Design review of the part built by this model. Coordinates are the model's own, in mm. Face numbers are marked on the shaded views. A direction names the side the tool comes from. Coordinates: 2 decimals unless noted, no trailing zeros. Loops run counter-clockwise (first coordinate to the right, second up) from the corner with the lowest first, then second, coordinate; pieces in that order, holes last. Notation, with made-up numbers: (-39, -14) -> (-15, -14) arc R5 ccw to (-15, -8) -> close; hole circle Ø1 at (34, 28.25). An arc over 180 degrees is marked (long way). Use CSV: the item, a comma, the result in double quotes.
```python
from build123d import *

# Parameters (mm, degrees)
ESQUISSE1_R                  = 4.25
ESQUISSE1_R_2                = 1.7
BOSS_EXTRU_1_DEPTH           = 5
ESQUISSE2_R                  = 3
ENL_V_MAT_EXTRU_1_DEPTH      = 3
BOSS_EXTRU_2_DEPTH           = 3
R_P_TITION_CIRCULAIRE1_DEPTH = 4
ESQUISSE4_R                  = 1
BOSS_EXTRU_3_DEPTH           = 2
R_P_TITION_CIRCULAIRE2_COUNT = 6
ENL_V_START                  = -1
ESQUISSE5_R                  = 3
ENL_V_MAT_EXTRU_2_DEPTH      = 1
CONG_1_R                     = 0.2
ESQUISSE6_R                  = 4.5
ESQUISSE6_R_2                = 3.5
ENL_V_MAT_EXTRU_3_DEPTH      = 1
CONG_2_R                     = 0.25
SCALE1_SCALE                 = 1.05


with BuildPart() as part:
    # Esquisse1 → Boss.-Extru.1 (new body)
    with BuildSketch(Plane.XY):
        Circle(ESQUISSE1_R)
        Circle(ESQUISSE1_R_2, mode=Mode.SUBTRACT)
    extrude(amount=BOSS_EXTRU_1_DEPTH)

    # Esquisse2 → Enlèv. mat.-Extru.1 (cut)
    with BuildSketch(Plane(origin=(0, 0, 0), x_dir=(-1, 0, 0), z_dir=(0, 0, -1))):
        Circle(ESQUISSE2_R)
    extrude(amount=-ENL_V_MAT_EXTRU_1_DEPTH, mode=Mode.SUBTRACT)

    # Esquisse3 → Boss.-Extru.2 (add)
    with BuildSketch(Plane(origin=(0, 0, 0), x_dir=(-1, 0, 0), z_dir=(0, 0, -1))):
        Polygon((-0.3, 3), (0, 2.6), (0.3, 3), align=None)
    extrude(amount=-BOSS_EXTRU_2_DEPTH)

    # Répétition circulaire1: read off the stored shape, not the designer's step
    # Répétition circulaire1 outline → Répétition circulaire1 (add)
    with BuildSketch(Plane.XY):
        with BuildLine():
            ThreePointArc((1.052468236, 2.80932565), (0.776457135, 2.897777479), (0.493198596, 2.959181499))
            Line((0.493198596, 2.959181499), (0.672929517, 2.511407148))
            Line((0.672929517, 2.511407148), (1.052468236, 2.80932565))
        make_face()
        with BuildLine():
            ThreePointArc((-0.493198596, 2.959181499), (-0.776457135, 2.897777479), (-1.052468236, 2.80932565))
            Line((-1.052468236, 2.80932565), (-0.672929517, 2.511407148))
            Line((-0.672929517, 2.511407148), (-0.493198596, 2.959181499))
        make_face()
        with BuildLine():
            ThreePointArc((-1.242285791, 2.730700645), (-1.5, 2.598076211), (-1.743713233, 2.441201376))
            Line((-1.743713233, 2.441201376), (-1.3, 2.25166605))
            Line((-1.3, 2.25166605), (-1.242285791, 2.730700645))
        make_face()
        with BuildLine():
            ThreePointArc((-1.906713263, 2.316127054), (-2.121320343, 2.121320343), (-2.316127054, 1.906713263))
            Line((-2.316127054, 1.906713263), (-1.838477631, 1.838477631))
            Line((-1.838477631, 1.838477631), (-1.906713263, 2.316127054))
        make_face()
        with BuildLine():
            ThreePointArc((-2.441201376, 1.743713233), (-2.598076211, 1.5), (-2.730700645, 1.242285791))
            Line((-2.730700645, 1.242285791), (-2.25166605, 1.3))
            Line((-2.25166605, 1.3), (-2.441201376, 1.743713233))
        make_face()
        with BuildLine():
            ThreePointArc((-2.809325651, 1.052468236), (-2.897777479, 0.776457135), (-2.959181499, 0.493198596))
            Line((-2.959181499, 0.493198596), (-2.511407148, 0.672929517))
            Line((-2.511407148, 0.672929517), (-2.809325651, 1.052468236))
        make_face()
        with BuildLine():
            ThreePointArc((-2.985999024, 0.289499268), (-3, 0), (-2.985999024, -0.289499268))
            Line((-2.985999024, -0.289499268), (-2.6, 0))
            Line((-2.6, 0), (-2.985999024, 0.289499268))
        make_face()
        with BuildLine():
            ThreePointArc((-2.959181499, -0.493198596), (-2.897777479, -0.776457135), (-2.809325651, -1.052468236))
            Line((-2.809325651, -1.052468236), (-2.511407148, -0.672929517))
            Line((-2.511407148, -0.672929517), (-2.959181499, -0.493198596))
        make_face()
        with BuildLine():
            ThreePointArc((-2.730700645, -1.242285791), (-2.598076211, -1.5), (-2.441201377, -1.743713233))
            Line((-2.441201377, -1.743713233), (-2.25166605, -1.3))
            Line((-2.25166605, -1.3), (-2.730700645, -1.242285791))
        make_face()
        with BuildLine():
            ThreePointArc((-2.316127055, -1.906713263), (-2.121320344, -2.121320344), (-1.906713263, -2.316127055))
            Line((-1.906713263, -2.316127055), (-1.838477631, -1.838477631))
            Line((-1.838477631, -1.838477631), (-2.316127055, -1.906713263))
        make_face()
        with BuildLine():
            ThreePointArc((-1.743713233, -2.441201377), (-1.5, -2.598076211), (-1.242285791, -2.730700645))
            Line((-1.242285791, -2.730700645), (-1.3, -2.25166605))
            Line((-1.3, -2.25166605), (-1.743713233, -2.441201377))
        make_face()
        with BuildLine():
            ThreePointArc((-1.052468236, -2.809325651), (-0.776457135, -2.897777479), (-0.493198596, -2.959181499))
            Line((-0.493198596, -2.959181499), (-0.672929517, -2.511407148))
            Line((-0.672929517, -2.511407148), (-1.052468236, -2.809325651))
        make_face()
        with BuildLine():
            ThreePointArc((-0.289499268, -2.985999024), (0, -3), (0.289499268, -2.985999024))
            Line((0.289499268, -2.985999024), (0, -2.6))
            Line((0, -2.6), (-0.289499268, -2.985999024))
        make_face()
        with BuildLine():
            ThreePointArc((0.493198596, -2.959181499), (0.776457135, -2.897777479), (1.052468236, -2.809325651))
            Line((1.052468236, -2.809325651), (0.672929517, -2.511407148))
            Line((0.672929517, -2.511407148), (0.493198596, -2.959181499))
        make_face()
        with BuildLine():
            ThreePointArc((1.242285791, -2.730700645), (1.5, -2.598076211), (1.743713233, -2.441201377))
            Line((1.743713233, -2.441201377), (1.3, -2.25166605))
            Line((1.3, -2.25166605), (1.242285791, -2.730700645))
        make_face()
        with BuildLine():
            ThreePointArc((1.906713263, -2.316127055), (2.121320344, -2.121320344), (2.316127055, -1.906713263))
            Line((2.316127055, -1.906713263), (1.838477631, -1.838477631))
            Line((1.838477631, -1.838477631), (1.906713263, -2.316127055))
        make_face()
        with BuildLine():
            ThreePointArc((2.441201377, -1.743713233), (2.598076211, -1.5), (2.730700645, -1.242285791))
            Line((2.730700645, -1.242285791), (2.25166605, -1.3))
            Line((2.25166605, -1.3), (2.441201377, -1.743713233))
        make_face()
        with BuildLine():
            ThreePointArc((2.809325651, -1.052468236), (2.897777479, -0.776457135), (2.959181499, -0.493198596))
            Line((2.959181499, -0.493198596), (2.511407148, -0.672929517))
            Line((2.511407148, -0.672929517), (2.809325651, -1.052468236))
        make_face()
        with BuildLine():
            ThreePointArc((2.985999024, -0.289499268), (3, 0), (2.985999024, 0.289499268))
            Line((2.985999024, 0.289499268), (2.6, 0))
            Line((2.6, 0), (2.985999024, -0.289499268))
        make_face()
        with BuildLine():
            ThreePointArc((2.959181499, 0.493198596), (2.897777479, 0.776457135), (2.809325651, 1.052468236))
            Line((2.809325651, 1.052468236), (2.511407148, 0.672929517))
            Line((2.511407148, 0.672929517), (2.959181499, 0.493198596))
        make_face()
        with BuildLine():
            ThreePointArc((2.730700645, 1.242285791), (2.598076211, 1.5), (2.441201376, 1.743713233))
            Line((2.441201376, 1.743713233), (2.25166605, 1.3))
            Line((2.25166605, 1.3), (2.730700645, 1.242285791))
        make_face()
        with BuildLine():
            ThreePointArc((2.316127054, 1.906713263), (2.121320343, 2.121320343), (1.906713263, 2.316127054))
            Line((1.906713263, 2.316127054), (1.838477631, 1.838477631))
            Line((1.838477631, 1.838477631), (2.316127054, 1.906713263))
        make_face()
        with BuildLine():
            ThreePointArc((1.743713233, 2.441201376), (1.5, 2.598076211), (1.242285791, 2.730700645))
            Line((1.242285791, 2.730700645), (1.3, 2.25166605))
            Line((1.3, 2.25166605), (1.743713233, 2.441201376))
        make_face()
    extrude(amount=R_P_TITION_CIRCULAIRE1_DEPTH)

    # Esquisse4 → Boss.-Extru.3 (add)
    with BuildSketch(Plane.XY.offset(5)):
        with BuildLine():
            Line((-1.95061736, 14.441692106), (-3.75, 6.495190528))
            Line((-3.75, 6.495190528), (-3.75, 2))
            Line((-3.75, 2), (0, 3.364888378))
            Line((0, 3.364888378), (3.75, 2))
            Line((3.75, 2), (3.75, 6.495190528))
            Line((3.75, 6.495190528), (1.95061736, 14.441692106))
            ThreePointArc((1.95061736, 14.441692106), (0, 16), (-1.95061736, 14.441692106))
        make_face()
        with Locations((0, 7.5)):
            Circle(ESQUISSE4_R, mode=Mode.SUBTRACT)
        with Locations((0, 10.5)):
            Circle(ESQUISSE4_R, mode=Mode.SUBTRACT)
        with Locations((0, 13.5)):
            Circle(ESQUISSE4_R, mode=Mode.SUBTRACT)
    boss_extru_3 = extrude(amount=-BOSS_EXTRU_3_DEPTH)

    # Répétition circulaire2: Boss.-Extru.3 ×6 about axis
    r_p_tition_circulaire2_axis = Axis((0, 0, 0), (0, 0, 1))
    for i in range(1, R_P_TITION_CIRCULAIRE2_COUNT):
        add(boss_extru_3.rotate(r_p_tition_circulaire2_axis, i * 360 / R_P_TITION_CIRCULAIRE2_COUNT))

    # Esquisse5 → Enlèv. mat.-Extru.2 (cut)
    with BuildSketch(Plane.XY.offset(5).offset(ENL_V_START)):
        Circle(ESQUISSE5_R)
    extrude(amount=ENL_V_MAT_EXTRU_2_DEPTH, mode=Mode.SUBTRACT)

    # Congé1
    cong_1_edges = [part.edges().sort_by_distance(p)[0] for p in [
        (-4.25, 0, 0),
    ]]
    fillet(cong_1_edges, radius=CONG_1_R)

    # Esquisse6 → Enlèv. mat.-Extru.3 (cut)
    with BuildSketch(Plane.XY.offset(5)):
        Circle(ESQUISSE6_R)
        Circle(ESQUISSE6_R_2, mode=Mode.SUBTRACT)
    extrude(amount=-ENL_V_MAT_EXTRU_3_DEPTH, mode=Mode.SUBTRACT)

    # Congé2
    cong_2_edges = [part.edges().sort_by_distance(p)[0] for p in [
        (-3, 0, 5),
        (-4.5, 0, 5),
        (-3.5, 0, 5),
    ]]
    fillet(cong_2_edges, radius=CONG_2_R - 0.0001)  # a hair under: the kernel refuses the full size


with BuildPart() as part_1:
    # Scale1: scaled about (0, 0, 3.681971043)
    add(part.part.scale(SCALE1_SCALE).moved(Location((0, 0, -0.184098552))))


solid = part_1.part
```
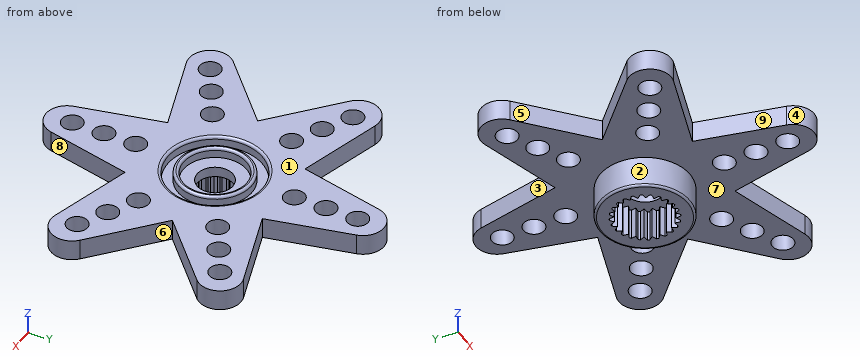
Item 1: Draft analysis for pull direction X (two halves, no side actions). For the marked faces 6, 7, 8 and 9, state which applies: pulls with the +X half, pulls with the -X half, needs draft (parallel to the pull), parting line crosses it, or undercut.
Checked values:
face 6,"pulls with the +X half"
face 7,"needs draft"
face 8,"undercut"
face 9,"undercut"
Item 2: Machinability: for the marked faces 1, 2, 3, 4 and 5, which of the approach directions +Z, -Z, +X, -X, +Y, -Y give a long, thin tool a straight path to every point of the face, cutting with its end or side? Answer none if there is none.
Checked values:
face 1,"+Z, +X, -X, +Y, -Y"
face 2,"-Z"
face 3,"+Z, -Z, +Y"
face 4,"+Z, -Z, -Y"
face 5,"+Z, -Z, -X"
Item 3: Clearance check with flat-ended pins moving along their axes: pin 1 (3.5 mm diameter, centred on x = 0, y = 7.875, fed in from +Z); pin 2 (1.5 mm diameter, centred on y = 3, z = 0.5, fed in from -X); pin 3 (1.5 mm diameter, centred on x = -9.5, z = 3.5, fed in from +Y); pin 4 (2.5 mm diameter, centred on x = 0, y = 14.175, fed in from -Z). State where each tip first meets the part, or that it passes through.
Checked values:
pin 1,"z = 5.07"
pin 2,"x = -3.85"
pin 3,"y = 8.78"
pin 4,"z = 2.97"
Item 4: To check wall thickness, follow line 1 along X through (y, z) = (4, 3.4); line 2 along Y through (x, z) = (3, 2.3); line 3 along Y through (x, z) = (-9, 4.5). State the ranges of each line that lie inside material, in increasing order.
Checked values:
line 1,"-12.2 to -7.87, -5.77 to 5.77, 7.87 to 12.2"
line 2,"-3.3 to -0.56, -0.2 to 0.2, 0.56 to 3.3"
line 3,"-8.39 to -6.41, -4.62 to -1.04, 1.04 to 4.62, 6.41 to 8.39"
Item 5: Add section A-A (y = 11.5). Give the boundary of the cut face in (x, z).
Checked values:
outline,"(-2.88, 2.97) -> (-0.94, 2.97) -> (-0.94, 5.07) -> (-2.88, 5.07) -> close; (0.94, 2.97) -> (2.88, 2.97) -> (2.88, 5.07) -> (0.94, 5.07) -> close"
